Build history of the part. All positions in model axes, mm. A direction names the side the tool comes from. Round coordinates to 2 decimals unless told otherwise and drop trailing zeros. Loops run counter-clockwise (first coordinate to the right, second up) from the corner with the lowest first, then second, coordinate; pieces in that order, holes last. Notation, with made-up numbers: (68, 81.5) - (99, 81.5) arc R31 ccw to (99, 115.5) - close; hole circle Ø11 at (23, 7.5). An arc over 180 degrees is marked (long way). Use a Markdown table: item, result.
Autodesk Inventor part; units mm, degrees
ref_plane "YZ Plane" through (0, 0, 0) normal (1, 0, 0) x (0, 1, 0)
ref_plane "XZ Plane" through (0, 0, 0) normal (0, 1, 0) x (-1, 0, 0)
ref_plane "XY Plane" through (0, 0, 0) normal (0, 0, 1) x (1, 0, 0)
sketch "Sketch1" plane through (0, 0, 0) normal (1, 0, 0) x (0, 1, 0)
  line L0 (-42.75, 165) -> (42.75, 165) construction
  line L1 (42.75, 165) -> (42.75, 0) construction
  line L2 (42.75, 0) -> (-42.75, 0) construction
  line L3 (-42.75, 0) -> (-42.75, 165) construction
  arc A0 (-32.6897, 172.419) -> (-50.4192, 155.1291) centre (-42.75, 165) ccw
  arc A1 (50.4158, 155.1265) -> (32.6897, 172.419) centre (42.75, 165) ccw
  arc A2 (-50.4296, 9.8627) -> (-32.6897, -7.419) centre (-42.75, 0) ccw
  arc A3 (32.6897, -7.419) -> (50.433, 9.8601) centre (42.75, 0) ccw
  line L4 (0, 0) -> (0, 165) construction
  line L5 (-19.1029, 0) -> (-19.1029, 82.5) construction
  line L6 (-42.75, 82.5346) -> (42.75, 82.5346) construction
  line L7 (-42.75, 82.5346) -> (-62.75, 82.5346) construction
  line L8 (42.75, 82.5346) -> (62.75, 82.5346) construction
  arc A4 (-62.75, 95.0346) -> (-62.75, 70.0346) centre (-62.75, 82.5346) ccw
  arc A5 (62.7626, 70.0346) -> (62.7374, 95.0346) centre (62.75, 82.5346) ccw
  circle A6 centre (-62.75, 82.5346) radius 3.5
  circle A7 centre (62.75, 82.5346) radius 3.5
  circle A8 centre (-42.75, 165) radius 3.5
  circle A9 centre (42.75, 165) radius 3.5
  circle A10 centre (-42.75, 0) radius 3.5
  circle A11 centre (42.75, 0) radius 3.5
  line L9 (42.75, 165) -> (33.9112, 173.8388) construction
  line L10 (-42.75, 165) -> (-33.9112, 173.8388) construction
  line L11 (42.75, 165) -> (51.5888, 156.1612) construction
  line L12 (-42.75, 165) -> (-51.5888, 156.1612) construction
  line L13 (-42.75, 0) -> (-51.5888, 8.8388) construction
  line L14 (-42.75, 0) -> (-33.9112, -8.8388) construction
  line L15 (42.75, 0) -> (33.9112, -8.8388) construction
  line L16 (42.75, 0) -> (51.5888, 8.8388) construction
  line L17 (-62.75, 82.5346) -> (-62.75, 95.0346) construction
  line L18 (-62.75, 82.5346) -> (-62.75, 70.0346) construction
  line L19 (62.75, 82.5346) -> (62.7374, 95.0346) construction
  line L20 (62.75, 82.5346) -> (62.7626, 70.0346) construction
  line L21 (-51.5888, 156.1612) -> (-62.75, 95.0346) construction
  line L22 (-33.9112, 173.8388) -> (33.9112, 173.8388) construction
  line L23 (51.5888, 156.1612) -> (62.7374, 95.0346) construction
  line L24 (62.7626, 70.0346) -> (51.5888, 8.8388) construction
  line L25 (33.9112, -8.8388) -> (-33.9112, -8.8388) construction
  line L26 (-51.5888, 8.8388) -> (-62.75, 70.0346) construction
  line L27 (-57.1694, 125.5979) -> (-39.4622, 122.3647) construction
  line L28 (57.1631, 125.5979) -> (39.4552, 122.3682) construction
  line L29 (-57.1694, 39.4367) -> (-39.4615, 42.6664) construction
  line L30 (57.1757, 39.4367) -> (39.4685, 42.6699) construction
  line L31 (0, -8.8388) -> (0, 7.1612)
  arc A12 (-33.9112, 173.8388) -> (33.9112, 173.8388) centre (0, 201.7753) ccw
  arc A13 (-62.75, 95.0346) -> (-51.5888, 156.1612) centre (-74.6924, 128.7974) ccw
  arc A14 (-51.5888, 8.8388) -> (-62.75, 70.0346) centre (-74.7509, 36.2301) ccw
  arc A15 (62.7626, 70.0346) -> (51.5888, 8.8388) centre (74.7585, 36.2263) ccw
  arc A16 (33.9112, -8.8388) -> (-33.9112, -8.8388) centre (0, -36.7753) ccw
  arc A17 (51.5888, 156.1612) -> (62.7374, 95.0346) centre (74.6848, 128.7936) ccw
  line L32 (-42.75, 99.1738) -> (-31.75, 99.1738) construction
  line L33 (42.75, 99.1738) -> (31.75, 99.1738) construction
  line L34 (0, 157.8388) -> (0, 7.1612) construction
  line L35 (-25.75, 165) -> (-25.75, 103.3033) construction
  line L36 (-31.75, 91.7175) -> (31.75, 91.7175)
  line L37 (31.75, 91.7175) -> (31.75, 73.7175)
  line L38 (31.75, 73.7175) -> (-31.75, 73.7175)
  line L39 (-31.75, 73.7175) -> (-31.75, 91.7175)
  line L40 (0, 142.2444) -> (-32.5269, 109.7175)
  line L41 (-32.5269, 109.7175) -> (32.5269, 109.7175)
  line L42 (32.5269, 109.7175) -> (0, 142.2444)
  line L43 (0, 23.1637) -> (-32.5, 55.7175)
  line L44 (-32.5, 55.7175) -> (32.5, 55.7175)
  line L45 (32.5, 55.7175) -> (0, 23.1637)
  circle A18 centre (0, 151.3388) radius 1
  circle A19 centre (25.75, 124.7175) radius 1
  circle A20 centre (-25.75, 124.7175) radius 1
  circle A21 centre (-25.75, 40.7175) radius 1
  circle A22 centre (25.75, 40.7175) radius 1
  dimension "d0" = 165
  dimension "d1" = 85.5
  dimension "d2" = 82.5
  dimension "d3" = 20
  dimension "d4" = 20
  dimension "d5" = 25
  dimension "d6" = 25
  dimension "d7" = 25
  dimension "d8" = 25
  dimension "d9" = 25
  dimension "d10" = 25
  dimension "d11" = 7
  dimension "d12" = 7
  dimension "d13" = 7
  dimension "d14" = 7
  dimension "d15" = 7
  dimension "d16" = 7
  dimension "d17" = 45
  dimension "d18" = 45
  dimension "d19" = 45
  dimension "d20" = 45
  dimension "d21" = 45
  dimension "d22" = 45
  dimension "d23" = 45
  dimension "d24" = 90
  dimension "d26" = 16
  dimension "d27" = 11
  dimension "d28" = 11
  dimension "d29" = 150.6777
  dimension "d30" = 61.6967
  dimension "d31" = 63.5
  dimension "d32" = 18
  dimension "d33" = 73.2825
  dimension "d34" = 31
  dimension "d35" = 46
  dimension "d36" = 46
  dimension "d37" = 65.0538
  dimension "d38" = 18
  dimension "d39" = 65
  dimension "d40" = 46
  dimension "d41" = 46
  dimension "d42" = 18
  dimension "d43" = 2
  dimension "d44" = 6.5
  dimension "d45" = 2
  dimension "d46" = 2
  dimension "d47" = 33
  dimension "d48" = 17
  dimension "d49" = 17
  dimension "d50" = 33
  dimension "d51" = 2
  dimension "d52" = 2
  dimension "d53" = 33
  dimension "d54" = 33
  dimension "d55" = 17
  dimension "d56" = 17
extrude "Extrusion1" add sketch "Sketch1" along normal blind 2 contours A12 A1 A17 A5 A15 A3 A16 A2 A14 A4 A13 A0
properties part number "BaseBawah"
Q1. Cut at A-A, the plane z = 45. List the corners of the cut face in (x, y).
Results found:
| item | result |
|---|---|
| outline | (0, -39.97) - (2, -39.97) - (2, -21.8) - (0, -21.8) - close; (0, 21.8) - (2, 21.8) - (2, 39.97) - (0, 39.97) - close |
Q2. Cut at C-C, the plane y = -42.75. List the corners of the cut face in (x, z), plus the area to 3 significant figures.
Results found:
| item | result |
|---|---|
| outline | (0, -12.5) - (2, -12.5) - (2, -3.5) - (0, -3.5) - close; (0, 3.5) - (2, 3.5) - (2, 20.02) - (0, 20.02) - close; (0, 52.44) - (2, 52.44) - (2, 112.6) - (0, 112.6) - close; (0, 144.99) - (2, 144.99) - (2, 161.5) - (0, 161.5) - close; (0, 168.5) - (2, 168.5) - (2, 177.5) - (0, 177.5) - close |
| area | 222 mm2 |
Q3. Which spindle directions (+Z, -Z, +X, -X, +Y, -Y) get a long thin tool onto all of the face, cutting with end or side? Do faces 1 (the face through (0.986, -0.542, 7.158)), 2 (the face through (0.986, -16.036, 126.209)). Say none if no direction does.
Results found:
| item | result |
|---|---|
| face 1 | -Z, +X, -X |
| face 2 | +X, -X |
Q4. Drop flat-ended pins along their axis: pin 1 (9 mm diameter, centred on y = 42.75, z = 165, fed in from -X); pin 2 (1 mm diameter, centred on x = 1, z = 83.5, fed in from +Y); pin 3 (1.2 mm diameter, centred on y = -25.75, z = 124.72, fed in from +X). Give the stop position or say it passes through.
Results found:
| item | result |
|---|---|
| pin 1 | stops at x = 0 |
| pin 2 | stops at y = 75.24 |
| pin 3 | passes through |
Q5. Cut at B-B, the plane x = 0.6. Count the separate pieces of the cut face and the enclosed holes in it, plus the area to 3 significant figures.
Results found:
| item | result |
|---|---|
| separate pieces | 1 |
| enclosed holes | 14 |
| area | 13,400 mm2 |
Q6. Probe line 1 (Z direction, x = 0.75, y = 0); line 2 (Y direction, x = 1.35, z = 41); line 3 (Y direction, x = 1.8, z = 40). List the from-to ranges inside material, lowest first.
Results found:
| item | result |
|---|---|
| line 1 | z = 7.16 to 23.16, 55.72 to 73.72, 91.72 to 109.72, 142.24 to 150.34, 152.34 to 157.84 |
| line 2 | y = -39.2 to -26.71, -24.79 to -17.81, 17.81 to 24.79, 26.71 to 39.2 |
| line 3 | y = -39.08 to -26.45, -25.05 to -16.81, 16.81 to 25.05, 26.45 to 39.08 |
Q7. Cut at D-D, the plane z = 165. List the corners of the cut face in (x, y).
Results found:
| item | result |
|---|---|
| outline | (0, -55.25) - (2, -55.25) - (2, -46.25) - (0, -46.25) - close; (0, -39.25) - (2, -39.25) - (2, -24.04) - (0, -24.04) - close; (0, 24.04) - (2, 24.04) - (2, 39.25) - (0, 39.25) - close; (0, 46.25) - (2, 46.25) - (2, 55.25) - (0, 55.25) - close |
Q8. Pull direction Y, two halves, no side cores. Call faces 3 (the face through (0.986, -46.247, -0.154)), 4 (the face through (0.99, -39.37, 122.88)), 5 (the face through (0.99, -63.51, 85.95)), 6 (the face through (0, -1, 105)): pulls with the +Y half, pulls with the -Y half, needs draft (parallel to the pull), parting line crosses it, or undercut.
Results found:
| item | result |
|---|---|
| face 3 | undercut |
| face 4 | pulls with the -Y half |
| face 5 | undercut |
| face 6 | needs draft |
